Could you check a few things on this drawing? It's one solid part, dimensions in mm from its lowest x, y, z. Give positions to 0.01 mm unless a question says otherwise; leave off trailing zeros. Order: outer loops, then holes, each group sorted by start corner. A loop starts at its lowest first (then second) coordinate and runs counter-clockwise, first axis right, second up. Notation, with made-up numbers: M -4,66 L 44,66 A30 cw 44,104 Z; hole C 13,21.5 d1. An arc over 180 degrees is marked long. Use one line per item in the form item = value. Start each with the question number.
1. We'd pull the mould along X, two halves only. Please class the marked faces 1 and 2: +X half, -X half, draft (parallel to the pull), parting line (faces both ways), or undercut.
2. I need wall thicknesses on L1, parallel to Y at x = 114, z = 7.5; L2, parallel to Z at x = 111, y = 56.5. Which ranges of each line are inside material? Lowest first, please.
3. I want a section at B-B, the plane x = 139.7. List the corners of the cut face in (y, z) for me, and give its area (3 significant figures).
4. I want a section at A-A, the plane z = 10. Count the separate pieces of the cut face and the enclosed holes in it, and give its area (3 significant figures).
5. I want a section at C-C, the plane y = 63.5. List the corners of the cut face in (x, z) for me.
6. I want a section at D-D, the plane x = 88.5. List the corners of the cut face in (y, z) for me.
7. Will this pin go through, and if not, where does the flat tip stop? P1, Ø6, axis at x = 40, z = 11.5, coming from the +Y side.
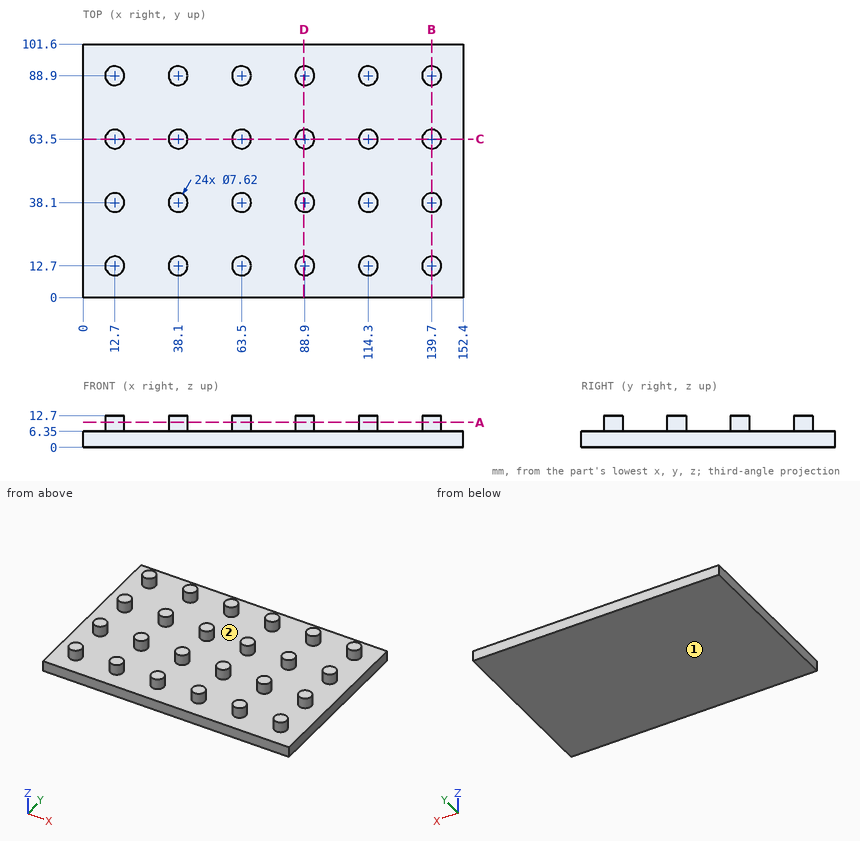
Check result:
q1.face_1 = draft
q1.face_2 = undercut
q2.L1 = 8.9 to 16.5, 34.3 to 41.9, 59.7 to 67.3, 85.1 to 92.7
q2.L2 = 0 to 6.35
q3.outline = M 0,0 L 101.6,0 L 101.6,6.35 L 92.71,6.35 L 92.71,12.7 L 85.09,12.7 L 85.09,6.35 L 67.31,6.35 L 67.31,12.7 L 59.69,12.7 L 59.69,6.35 L 41.91,6.35 L 41.91,12.7 L 34.29,12.7 L 34.29,6.35 L 16.51,6.35 L 16.51,12.7 L 8.89,12.7 L 8.89,6.35 L 0,6.35 Z
q3.area = 839 mm2
q4.separate_pieces = 24
q4.enclosed_holes = 0
q4.area = 1,090 mm2
q5.outline = M 0,0 L 152.4,0 L 152.4,6.35 L 143.51,6.35 L 143.51,12.7 L 135.89,12.7 L 135.89,6.35 L 118.11,6.35 L 118.11,12.7 L 110.49,12.7 L 110.49,6.35 L 92.71,6.35 L 92.71,12.7 L 85.09,12.7 L 85.09,6.35 L 67.31,6.35 L 67.31,12.7 L 59.69,12.7 L 59.69,6.35 L 41.91,6.35 L 41.91,12.7 L 34.29,12.7 L 34.29,6.35 L 16.51,6.35 L 16.51,12.7 L 8.89,12.7 L 8.89,6.35 L 0,6.35 Z
q6.outline = M 0,0 L 101.6,0 L 101.6,6.35 L 92.69,6.35 L 92.69,12.7 L 85.11,12.7 L 85.11,6.35 L 67.29,6.35 L 67.29,12.7 L 59.71,12.7 L 59.71,6.35 L 41.89,6.35 L 41.89,12.7 L 34.31,12.7 L 34.31,6.35 L 16.49,6.35 L 16.49,12.7 L 8.91,12.7 L 8.91,6.35 L 0,6.35 Z
q7.P1 = 92.71
